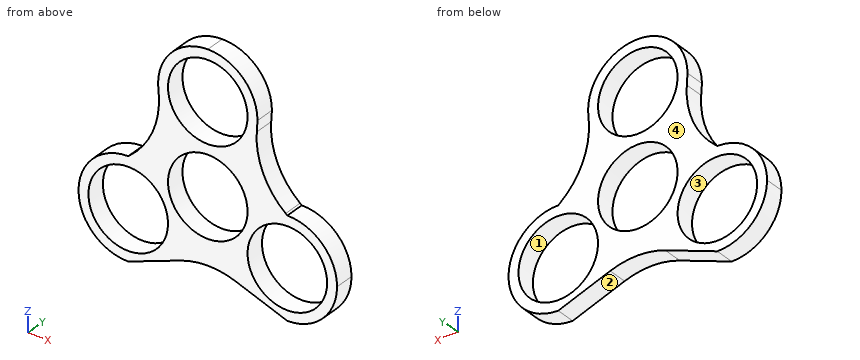
from build123d import *

# Parameters (mm, degrees)
F0_R     = 12.7
F1_DEPTH = 3.175


with BuildPart() as f1:
    # F0 (on Front) → F1 (new body, symmetric)
    with BuildSketch(Plane.XZ):
        with BuildLine():
            ThreePointArc((-41.275, 0), (-36.62532, -11.22532), (-25.4, -15.875))
            Line((-25.4, -15.875), (-8.814026, -9.738189))
            ThreePointArc((-8.814026, -9.738189), (0, -8.15988), (8.814026, -9.738189))
            Line((8.814026, -9.738189), (25.4, -15.875))
            ThreePointArc((25.4, -15.875), (36.62532, -11.22532), (41.275, 0))
            ThreePointArc((41.275, 0), (36.62532, 11.22532), (25.4, 15.875))
            Line((25.4, 15.875), (24.860597, 16.31807))
            ThreePointArc((24.860597, 16.31807), (17.667983, 25.866743), (15.639876, 37.647984))
            Line((15.639876, 37.647984), (15.875, 41.148))
            ThreePointArc((15.875, 41.148), (11.22532, 52.37332), (0, 57.023))
            ThreePointArc((0, 57.023), (-11.22532, 52.37332), (-15.875, 41.148))
            Line((-15.875, 41.148), (-15.639876, 37.647984))
            ThreePointArc((-15.639876, 37.647984), (-17.667983, 25.866743), (-24.860597, 16.31807))
            Line((-24.860597, 16.31807), (-25.4, 15.875))
            ThreePointArc((-25.4, 15.875), (-36.62532, 11.22532), (-41.275, 0))
        make_face()
        with Locations((-25.4, 0)):
            Circle(F0_R, mode=Mode.SUBTRACT)
        with Locations((25.4, 0)):
            Circle(F0_R, mode=Mode.SUBTRACT)
        with Locations((0, 12.573)):
            Circle(F0_R, mode=Mode.SUBTRACT)
        with Locations((0, 41.148)):
            Circle(F0_R, mode=Mode.SUBTRACT)
    extrude(amount=F1_DEPTH, both=True)


solid = f1.part
The model under review builds one solid part; all positions refer to its coordinate system, in mm. Face numbers are marked on the shaded views. Round coordinates to 2 decimals unless told otherwise and drop trailing zeros. Order: outer loops, then holes, each group sorted by start corner. A loop starts at its lowest first (then second) coordinate and runs counter-clockwise, first axis right, second up. Notation, with made-up numbers: (47.25, 27) -> (92.25, 27) arc R8 cw to (92.25, 34) -> close; hole circle Ø9 at (83, 84.5). An arc over 180 degrees is marked (long way). Return JSON: item names as keys, results as strings.
1. For L1, parallel to Z at x = -25.4, y = 1 (3 decimals); L2, parallel to Z at x = 1.5, y = -1; L3, parallel to X at y = -1.5, z = 2, list the stretches that pass through material, from the lowest coordinate up. Write a range as [from, to].
Answer block:
{"L1": "z = [-15.875, -12.7], [12.7, 15.875]", "L2": "z = [-8.2, -0.04], [25.18, 28.54], [53.76, 56.95]", "L3": "x = [-41.15, -37.94], [-12.86, -7.04], [7.04, 12.86], [37.94, 41.15]"}
2. Take a section at D-D (y = -0.5). State how many separate pieces and enclosed holes the cut face has, then the cut area to 3 significant figures.
Answer block:
{"separate pieces": "1", "enclosed holes": "4", "area": "1,450 mm²"}
3. Take a section at C-C (z = 29.5). Write out the cut boundary in (x, y) (3 decimals).
Answer block:
{"outline": "(-16.414, -3.175) -> (-5.061, -3.175) -> (-5.061, 3.175) -> (-16.414, 3.175) -> close; (5.061, -3.175) -> (16.414, -3.175) -> (16.414, 3.175) -> (5.061, 3.175) -> close"}
4. Take a section at B-B (z = 7.5). Write out the cut boundary in (x, y) (3 decimals).
Answer block:
{"outline": "(-39.392, -3.175) -> (-35.649, -3.175) -> (-35.649, 3.175) -> (-39.392, 3.175) -> close; (-15.151, -3.175) -> (-11.643, -3.175) -> (-11.643, 3.175) -> (-15.151, 3.175) -> close; (11.643, -3.175) -> (15.151, -3.175) -> (15.151, 3.175) -> (11.643, 3.175) -> close; (35.649, -3.175) -> (39.392, -3.175) -> (39.392, 3.175) -> (35.649, 3.175) -> close"}
5. Take a section at A-A (x = 27). Write out the cut boundary in (y, z) (3 decimals), then the cut area to 3 significant figures.
Answer block:
{"outline": "(-3.175, -15.794) -> (3.175, -15.794) -> (3.175, -12.599) -> (-3.175, -12.599) -> close; (-3.175, 12.599) -> (3.175, 12.599) -> (3.175, 15.794) -> (-3.175, 15.794) -> close", "area": "40.6 mm²"}
6. Insertion check: P1, Ø12, axis at x = -27, z = 38.5, coming from the -Y side; P2, Ø2, axis at y = -0.5, z = 36.5, coming from the +X side; P3, Ø1.5, axis at x = -18, y = 1, coming from the -Z side; P4, Ø1.5, axis at y = 1.5, z = 7, coming from the -X side. Each pin has a flat end and moves straight along its axis. Give the tip position at first contact, or say it passes through.
Answer block:
{"P1": "passes through", "P2": "stops at x = 15.63", "P3": "stops at z = -13.41", "P4": "stops at x = -39.99"}
7. The part is to be moulded in two halves that separate along Z. For the marked faces 1, 2, 3 and 4, say which applies: +Z half, -Z half, draft (parallel to the pull), parting line (faces both ways), or undercut.
Answer block:
{"face 1": "undercut", "face 2": "-Z half", "face 3": "undercut", "face 4": "draft"}
